```python
from build123d import *

# Parameters (mm, degrees)
SKETCH1_W           = 736.6
SKETCH1_H           = 736.6
BOSS_EXTRUDE1_DEPTH = 863.6
SKETCH2_W           = 685.8
SKETCH2_H           = 25.4
BOSS_EXTRUDE2_DEPTH = 25.4


with BuildPart() as part:
    # Sketch1 → Boss-Extrude1 (new body)
    with BuildSketch(Plane(origin=(0, 0, 0), x_dir=(1, 0, 0), z_dir=(0, 1, 0))):
        Rectangle(SKETCH1_W, SKETCH1_H)
    extrude(amount=BOSS_EXTRUDE1_DEPTH)

    # Sketch2 → Boss-Extrude2 (add)
    with BuildSketch(Plane.XY.offset(368.3)):
        with Locations((0, 749.3)):
            Rectangle(SKETCH2_W, SKETCH2_H)
        with Locations((0, 495.3)):
            Rectangle(SKETCH2_W, SKETCH2_H)
        with Locations((0, 139.7)):
            Rectangle(SKETCH2_W, SKETCH2_H)
    extrude(amount=BOSS_EXTRUDE2_DEPTH)


solid = part.part
```
The listing builds one solid part. Answer for the finished solid, in the listing's coordinates (mm). A direction names the side the tool comes from. Give positions to 0.01 mm unless a question says otherwise; leave off trailing zeros. Loops run counter-clockwise (first coordinate to the right, second up) from the corner with the lowest first, then second, coordinate; pieces in that order, holes last. Notation, with made-up numbers: (67.5, -21) - (125.5, -21) arc R20 cw to (125.5, 2) - close; hole circle Ø1 at (-32, -12). An arc over 180 degrees is marked (long way). Return JSON: item names as keys, results as strings. Group by question number.
1. Determine the mould class of faces 6 (the flat face through (-342.9, 495, 381)), 7 (the flat face through (-5, 426, 368.3)), 8 (the flat face through (-5, 127, 381)) for opening direction Y: pulls with the +Y half, pulls with the -Y half, needs draft (parallel to the pull), parting line crosses it, or undercut.
2. Which of the six approach directions +Z, -Z, +X, -X, +Y, -Y give full straight-line access (tool end or side, diameter ignored) to faces 1 (the flat face through (-342.9, 140, 381)), 2 (the flat face through (-5, 762, 381)), 3 (the flat face through (-5, 749, 393.7)), 4 (the flat face through (-5, 152.4, 381)), 5 (the flat face through (342.9, 140, 381))?
3. Find section B-B (y = 418). Write down the section's boundary in (x, z).
4. Given pin 1 Ø12.5 at (x, z) = (-27, 377) entering from -Y; pin 2 Ø12.5 at (x, z) = (51, 382.5) entering from +Y; pin 3 Ø7.5 at (y, z) = (749.5, 380) entering from -X, each flat-ended and moving along its own axis, determine where each tip first touches the part or whether it passes through.
5. A straight line is drawn through the part: line 1 (Z direction, x = 198.5, y = 83). Find the intervals that lie inside material, in ascending order. Write a range as [from, to].
6. Find section A-A (x = -303). Write down the section's boundary in (y, z).
Verdict:
{
 "1": {"face 6": "needs draft", "face 7": "undercut", "face 8": "pulls with the -Y half"},
 "2": {"face 1": "+Z, -X, +Y, -Y", "face 2": "+Z, +X, -X, +Y", "face 3": "+Z, +X, -X, +Y, -Y", "face 4": "+Z, +X, -X", "face 5": "+Z, +X, +Y, -Y"},
 "3": {"outline": "(-368.3, -368.3) - (368.3, -368.3) - (368.3, 368.3) - (-368.3, 368.3) - close"},
 "4": {"pin 1": "stops at y = 127", "pin 2": "stops at y = 762", "pin 3": "stops at x = -342.9"},
 "5": {"line 1": "z = [-368.3, 368.3]"},
 "6": {"outline": "(0, -368.3) - (863.6, -368.3) - (863.6, 368.3) - (762, 368.3) - (762, 393.7) - (736.6, 393.7) - (736.6, 368.3) - (508, 368.3) - (508, 393.7) - (482.6, 393.7) - (482.6, 368.3) - (152.4, 368.3) - (152.4, 393.7) - (127, 393.7) - (127, 368.3) - (0, 368.3) - close"}
}
